```python
from build123d import *

# Parameters (mm, degrees)
SKETCH1_W           = 30
SKETCH1_H           = 34
BOSS_EXTRUDE1_DEPTH = 3
SKETCH2_W           = 30
SKETCH2_H           = 8
BOSS_EXTRUDE2_DEPTH = 4
CUT_EXTRUDE2_DEPTH  = 30
FILLET4_R           = 0.1
FILLET5_R           = 0.1
FILLET6_R           = 0.1
FILLET7_R           = 0.1
SKETCH5_R           = 1.5
CUT_EXTRUDE3_DEPTH  = 30
SKETCH7_W           = 30
SKETCH7_H           = 10
BOSS_EXTRUDE3_DEPTH = 2


with BuildPart() as part:
    # Sketch1 → Boss-Extrude1 (new body)
    with BuildSketch(Plane(origin=(0, 0, 0), x_dir=(1, 0, 0), z_dir=(0, 1, 0))):
        Rectangle(SKETCH1_W, SKETCH1_H)
    extrude(amount=BOSS_EXTRUDE1_DEPTH)

    # Sketch2 → Boss-Extrude2 (add)
    with BuildSketch(Plane(origin=(0, 3, 0), x_dir=(1, 0, 0), z_dir=(0, 1, 0))):
        with Locations((0, -13)):
            Rectangle(SKETCH2_W, SKETCH2_H)
        with Locations((0, 13)):
            Rectangle(SKETCH2_W, SKETCH2_H)
    extrude(amount=BOSS_EXTRUDE2_DEPTH)

    # Sketch4 → Cut-Extrude2 (cut)
    with BuildSketch(Plane(origin=(15, 0, 0), x_dir=(0, 0, -1), z_dir=(1, 0, 0))):
        Polygon((-9, 3), (-13, 3), (-9, 7), align=None)
        Polygon((9, 3), (13, 3), (9, 7), align=None)
    extrude(amount=-CUT_EXTRUDE2_DEPTH, mode=Mode.SUBTRACT)

    # Fillet4
    fillet4_edges = [part.edges().sort_by_distance(p)[0] for p in [
        (0, 7, 9),
    ]]
    fillet(fillet4_edges, radius=FILLET4_R)

    # Fillet5
    fillet5_edges = [part.edges().sort_by_distance(p)[0] for p in [
        (0, 3, 13),
    ]]
    fillet(fillet5_edges, radius=FILLET5_R)

    # Fillet6
    fillet6_edges = [part.edges().sort_by_distance(p)[0] for p in [
        (0, 3, -13),
    ]]
    fillet(fillet6_edges, radius=FILLET6_R)

    # Fillet7
    fillet7_edges = [part.edges().sort_by_distance(p)[0] for p in [
        (0, 7, -9),
    ]]
    fillet(fillet7_edges, radius=FILLET7_R)

    # Sketch5 → Cut-Extrude3 (cut)
    with BuildSketch(Plane(origin=(0, 7, 0), x_dir=(1, 0, 0), z_dir=(0, 1, 0))):
        with Locations(Location((-12, 14, 0), (0, 0, 270))):
            Circle(SKETCH5_R)
        with Locations(Location((12, 14, 0), (0, 0, 270))):
            Circle(SKETCH5_R)
        with Locations(Location((-12, -14, 0), (0, 0, 270))):
            Circle(SKETCH5_R)
        with Locations(Location((12, -14, 0), (0, 0, 270))):
            Circle(SKETCH5_R)
    extrude(amount=-CUT_EXTRUDE3_DEPTH, mode=Mode.SUBTRACT)

    # Sketch7 → Boss-Extrude3 (add)
    with BuildSketch(Plane(origin=(0, 3, 0), x_dir=(1, 0, 0), z_dir=(0, 1, 0))):
        Rectangle(SKETCH7_W, SKETCH7_H)
    extrude(amount=BOSS_EXTRUDE3_DEPTH)


solid = part.part
```
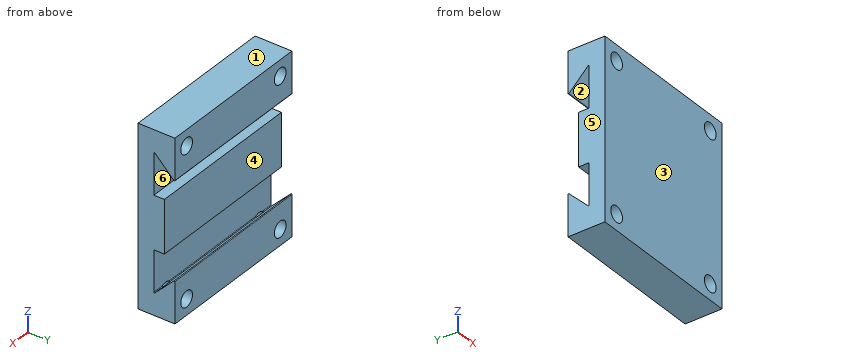
The listing builds one solid part. Answer for the finished solid, in the listing's coordinates (mm). Face numbers are marked on the shaded views. A direction names the side the tool comes from. Give positions to 0.01 mm unless a question says otherwise; leave off trailing zeros. Write each loop counter-clockwise with the first axis right and the second up, starting at its lowest first coordinate (ties: lowest second). Pieces come first, ordered by that corner, then holes. Notation, with made-up numbers: (-40, 17) - (-13, 17) arc R34 cw to (-13, 51) - close; hole circle Ø7 at (83, 23). An arc over 180 degrees is marked (long way). Use one line per item in the form item = value. Start each with the question number.
1) Find section A-A on x = 12. Determine the outline of the cut face in (y, z), plus the area to 3 significant figures.
2) The mould has two halves that part along Y. Classify the marked faces 1, 2 and 3: pulls with the +Y half, pulls with the -Y half, needs draft (parallel to the pull), parting line crosses it, or undercut.
3) Consider line 1 along X through (y, z) = (1.75, 14); line 2 along Y through (x, z) = (14.5, 11); line 3 along Z through (x, y) = (-7, 5.5). Determine where each line is inside the solid, lowest interval first. Write a range as from..to.
4) A tool of negligible diameter and unlimited length cuts with its end or side. For the marked faces 4, 5 and 6, from which of +Z, -Z, +X, -X, +Y, -Y can it reach the whole face along a straight path? Write none if from no direction.
5) Find section B-B on y = 4. Determine the outline of the cut face in (x, z), plus the area to 3 significant figures.
6) Find section D-D on z = -14. Determine the outline of the cut face in (x, y).
7) Flat-ended cylindrical pins translate along their axes: pin 1 Ø3 at (y, z) = (5.5, -6.5) entering from +X; pin 2 Ø2 at (x, z) = (-4, -3) entering from +Y. Find the tip coordinate at first contact, or state that the pin passes through.
8) Find section C-C on z = 12. Determine the outline of the cut face in (x, y), plus the area to 3 significant figures.
Geometry results:
q1.outline = (0, -17) - (7, -17) - (7, -15.5) - (0, -15.5) - close; (0, -12.5) - (3, -12.5) - (3, -5) - (5, -5) - (5, 5) - (3, 5) - (3, 12.5) - (0, 12.5) - close; (0, 15.5) - (7, 15.5) - (7, 17) - (0, 17) - close; (3.5, -12.5) - (7, -12.5) - (7, -9.24) arc R0.1 ccw to (6.83, -9.17) - close; (3.5, 12.5) - (6.83, 9.17) arc R0.1 ccw to (7, 9.24) - (7, 12.5) - close
q1.area = 128 mm2
q2.face_1 = needs draft
q2.face_2 = undercut
q2.face_3 = pulls with the -Y half
q3.line_1 = -15..-13.5, -10.5..10.5, 13.5..15
q3.line_2 = 0..3, 5..7
q3.line_3 = -17..-10.5, 10.5..17
q4.face_4 = +X, -X, +Y
q4.face_5 = +Z, -Z, -X, +Y, -Y
q4.face_6 = +X, -X
q5.outline = (-15, -17) - (15, -17) - (15, -12) - (-15, -12) - close; (-15, -5) - (15, -5) - (15, 5) - (-15, 5) - close; (-15, 12) - (15, 12) - (15, 17) - (-15, 17) - close; hole circle Ø3 at (-12, -14); hole circle Ø3 at (-12, 14); hole circle Ø3 at (12, -14); hole circle Ø3 at (12, 14)
q5.area = 572 mm2
q6.outline = (-15, 0) - (-13.5, 0) - (-13.5, 7) - (-15, 7) - close; (-10.5, 0) - (10.5, 0) - (10.5, 7) - (-10.5, 7) - close; (13.5, 0) - (15, 0) - (15, 7) - (13.5, 7) - close
q7.pin_1 = through
q7.pin_2 = 5
q8.outline = (-15, 0) - (15, 0) - (15, 3) - (-15, 3) - close; (-15, 4) - (15, 4) - (15, 7) - (-15, 7) - close
q8.area = 180 mm2
